```python
from build123d import *


with BuildPart() as part:
    # Sketch1 → Revolve1 (revolve)
    with BuildSketch(Plane.XY):
        with BuildLine():
            Line((1.5, 30), (26.5, 30))
            ThreePointArc((26.5, 30), (27.560660172, 30.439339828), (28, 31.5))
            Line((28, 31.5), (28, 36.35))
            ThreePointArc((28, 36.35), (26.217439951, 36.360351084), (24.439151002, 36.484108463))
            ThreePointArc((24.439151002, 36.484108463), (19.996363113, 36.996457171), (15.617923853, 37.907574657))
            Line((15.617923853, 37.907574657), (12.382076147, 37.907574657))
            ThreePointArc((12.382076147, 37.907574657), (8.003636887, 36.996457171), (3.560848998, 36.484108463))
            ThreePointArc((3.560848998, 36.484108463), (1.782560049, 36.360351084), (0, 36.35))
            Line((0, 36.35), (0, 31.5))
            ThreePointArc((0, 31.5), (0.439339828, 30.439339828), (1.5, 30))
        make_face()
    revolve(axis=Axis((28, 0, 0), (-1, 0, 0)))


solid = part.part
```
The listing builds one solid part. Answer for the finished solid, in the listing's coordinates (mm). Round coordinates to 2 decimals unless told otherwise and drop trailing zeros. Write each loop counter-clockwise with the first axis right and the second up, starting at its lowest first coordinate (ties: lowest second). Pieces come first, ordered by that corner, then holes. Notation, with made-up numbers: (-38.75, -37.75) -> (-29.75, -37.75) arc R7 ccw to (-29.75, -31.75) -> close; hole circle Ø1 at (-3, 12). An arc over 180 degrees is marked (long way). Answer as a JSON object with one key per item and string values. Group by question number.
Q1. Section C-C (x = 10.75) is taken. Write down the section's boundary in (y, z).
Q2. Straight lines are drawn through the part: line 1 along Z through (x, y) = (14.5, -1); line 2 along Y through (x, z) = (12.5, 0); line 3 along Z through (x, y) = (11, 0). For each, find the intervals that lie inside material, in ascending order.
Q3. Determine the mould class of faces 1 (the face through (14.18, -29.97, -1.32)), 2 (the face through (28, 11, -30)), 3 (the face through (13.977, 36.157, -11.386)) for opening direction Y: pulls with the +Y half, pulls with the -Y half, needs draft (parallel to the pull), parting line crosses it, or undercut.
Q4. Each of these flat-tipped pins is pushed along its axis until it touches: pin 1 Ø12 at (x, y) = (19.5, -28) entering from -Z; pin 2 Ø10 at (x, y) = (19, 5.5) entering from -Z; pin 3 Ø1 at (x, y) = (19.5, 3.5) entering from +Z. Where does it stop, or does it pass through?
Q5. Section A-A (y = 0) is taken. Write down the section's boundary in (x, z), plus the area to 3 significant figures.
Check values:
{
 "1": {"outline": "circle Ø75.04 at (0, 0); hole circle Ø60 at (0, 0)"},
 "2": {"line 1": "-37.89 to -29.98, 29.98 to 37.89", "line 2": "-37.91 to -30, 30 to 37.91", "line 3": "-37.58 to -30, 30 to 37.58"},
 "3": {"face 1": "undercut", "face 2": "needs draft", "face 3": "parting line crosses it"},
 "4": {"pin 1": "z = -30.07", "pin 2": "z = -37.86", "pin 3": "z = 37.01"},
 "5": {"outline": "(0, -36.35) arc R28 cw to (3.56, -36.48) arc R49.52 cw to (12.38, -37.91) -> (15.62, -37.91) arc R49.52 cw to (24.44, -36.48) arc R28 cw to (28, -36.35) -> (28, -31.5) arc R1.5 ccw to (26.5, -30) -> (1.5, -30) arc R1.5 ccw to (0, -31.5) -> close; (0, 31.5) arc R1.5 ccw to (1.5, 30) -> (26.5, 30) arc R1.5 ccw to (28, 31.5) -> (28, 36.35) arc R28 cw to (24.44, 36.48) arc R49.52 cw to (15.62, 37.91) -> (12.38, 37.91) arc R49.52 cw to (3.56, 36.48) arc R28 cw to (0, 36.35) -> close", "area": "389 mm^2"}
}
